Part model, mm, in its own coordinate system. A direction names the side the tool comes from. Give positions to 0.01 mm unless a question says otherwise; leave off trailing zeros. Order: outer loops, then holes, each group sorted by start corner. A loop starts at its lowest first (then second) coordinate and runs counter-clockwise, first axis right, second up.
1. Slice it at C-C on x = 0. Give the number of separate pieces and of enclosed holes in the cut face, and give its area (3 significant figures).
2. Slice it at D-D on z = -2. List the corners of the cut face in (x, y), and give its area (3 significant figures).
3. Slice it at B-B on y = 1. List the corners of the cut face in (x, z), and give its area (3 significant figures).
4. Mould opens along X. For faces 1 (the cylindrical face through (-1.29, -7.514, -2.024)), 2 (the flat face through (-16, 2, -4)), 3 (the cylindrical face through (-2.21, 2.03, -0.42)) say: +X half, -X half, draft (parallel to the pull), parting line (faces both ways), or undercut.
5. Slice it at A-A on z = -8. List the corners of the cut face in (x, y).
6. Probe line 1 (Z direction, x = 0, y = 5); line 2 (Y direction, x = -7, z = 2); line 3 (Z direction, x = 0, y = -6.75). List the from-to ranges inside material, lowest first.
7. Drop flat-ended pins along their axis: pin 1 Ø3 at (x, z) = (-23, -7.5) entering from +Y; pin 2 Ø6 at (y, z) = (-5.5, -4.5) entering from -X; pin 3 Ø6 at (x, z) = (2, -5.5) entering from +Y. Give the stop position or say it passes through.
8. Which spindle directions (+Z, -Z, +X, -X, +Y, -Y) get a long thin tool onto all of the face, cutting with end or side? Do faces 4 (the flat face through (-4, 0, 5)), 5 (the flat face through (-2, -6.5, 2)), 6 (the flat face through (0, 8.5, 2)), 7 (the flat face through (2, 6.5, 2)), 8 (the flat face through (-3, 3, -6)). Say none if no direction does.
from build123d import *

# Parameters (mm, degrees)
BOSS_EXTRUDE1_DEPTH            = 5
BOSS_EXTRUDE1_DEPTH_BACK       = 6
SKETCH2_R                      = 6
CUT_EXTRUDE1_REACH             = 14.01
SKETCH3_R                      = 3
CUT_EXTRUDE1_DIRECTION_2_REACH = 14.01
SKETCH4_R                      = 1.6
CUT_EXTRUDE4_DEPTH             = 17
BOSS_EXTRUDE2_DEPTH            = 2
BOSS_EXTRUDE2_DEPTH_BACK       = 2
SKETCH5_R                      = 1.35
FILLET1_R                      = 2
FILLET2_R                      = 1


with BuildPart() as part:
    # Sketch1 → Revolve1 (revolve)
    with BuildSketch(Plane.XY, mode=Mode.PRIVATE) as revolve1_sk:
        Polygon((1.6, -8.5), (1.6, 8.5), (2.4, 8.5), (2.4, 6.5), (4, 6.5), (4, -6.5), (2.4, -6.5), (2.4, -8.5), align=None)
    revolve(revolve1_sk.sketch.rotate(Axis((0, 9.772747413, 0), (0, -1, 0)), 180), axis=Axis((0, 9.772747413, 0), (0, -1, 0)))

    # Sketch2 → Boss-Extrude1 (add, two sides: drawn at the far end of the back side and taken through both)
    with BuildSketch(Plane.XY.offset(-BOSS_EXTRUDE1_DEPTH_BACK)):
        Circle(SKETCH2_R)
    extrude(amount=BOSS_EXTRUDE1_DEPTH + BOSS_EXTRUDE1_DEPTH_BACK)

    # Sketch3 → Cut-Extrude1 (cut, up to next)
    with BuildSketch(Plane.XY, mode=Mode.PRIVATE) as cut_extrude1_sk1:
        Circle(SKETCH3_R)
    cut_extrude1_tool1 = extrude(cut_extrude1_sk1.sketch, amount=-CUT_EXTRUDE1_REACH, mode=Mode.PRIVATE) & part.part
    add(cut_extrude1_tool1.solids().sort_by_distance((0, 0, 0))[0], mode=Mode.SUBTRACT)

    # Sketch3 → Cut-Extrude1 direction 2 (cut, up to next)
    with BuildSketch(Plane.XY, mode=Mode.PRIVATE) as cut_extrude1_direction_2_sk1:
        Circle(SKETCH3_R)
    cut_extrude1_direction_2_tool1 = extrude(cut_extrude1_direction_2_sk1.sketch, amount=CUT_EXTRUDE1_DIRECTION_2_REACH, mode=Mode.PRIVATE) & part.part
    add(cut_extrude1_direction_2_tool1.solids().sort_by_distance((0, 0, 0))[0], mode=Mode.SUBTRACT)

    # Sketch4 → Cut-Extrude4 (cut)
    with BuildSketch(Plane(origin=(0, 8.5, 0), x_dir=(1, 0, 0), z_dir=(0, 1, 0))):
        with Locations(Location((0, 0, 0), (0, 0, 180))):
            Circle(SKETCH4_R)
    extrude(amount=-CUT_EXTRUDE4_DEPTH, mode=Mode.SUBTRACT)

    # Sketch5 → Boss-Extrude2 (add, two sides: drawn at the far end of the back side and taken through both)
    with BuildSketch(Plane(origin=(0, 0, 0), x_dir=(1, 0, 0), z_dir=(0, 1, 0)).offset(-BOSS_EXTRUDE2_DEPTH_BACK)):
        with BuildLine():
            Line((-6, -5), (-10, -5))
            Line((-10, -5), (-25.5, 4))
            ThreePointArc((-25.5, 4), (-29.5, 8), (-25.5, 12))
            Line((-25.5, 12), (-23, 12))
            Line((-23, 12), (-8, 6))
            Line((-8, 6), (-6, 6))
            Line((-6, 6), (-3, 6))
            Line((-3, 6), (-3, -5))
            Line((-3, -5), (-6, -5))
        make_face()
        with Locations(Location((-25.5, 8, 0), (0, 0, 270))):
            Circle(SKETCH5_R, mode=Mode.SUBTRACT)
    extrude(amount=BOSS_EXTRUDE2_DEPTH + BOSS_EXTRUDE2_DEPTH_BACK)

    # Fillet1
    fillet1_edges = [part.edges().sort_by_distance(p)[0] for p in [
        (-5.656854249, 2, -0.5),
        (-5.656854249, -2, -0.5),
    ]]
    fillet(fillet1_edges, radius=FILLET1_R)

    # Fillet2
    fillet2_edges = [part.edges().sort_by_distance(p)[0] for p in [
        (-10, 0, 5),
        (-25.5, 0, -4),
        (-23, 0, -12),
        (-8, 0, -6),
    ]]
    fillet(fillet2_edges, radius=FILLET2_R)


solid = part.part
Data:
1. separate pieces: 4
1. enclosed holes: 0
1. area: 58.0 mm2
2. outline: (-22.06, -2) - (-6.93, -2) arc R2 cw to (-5.2, -3) arc R6 ccw to (-3.46, -4.9) - (-3.46, -6.5) - (-1.33, -6.5) - (-1.33, -8.5) - (1.33, -8.5) - (1.33, -6.5) - (3.46, -6.5) - (3.46, -4.9) arc R6 ccw to (3.46, 4.9) - (3.46, 6.5) - (1.33, 6.5) - (1.33, 8.5) - (-1.33, 8.5) - (-1.33, 6.5) - (-3.46, 6.5) - (-3.46, 4.9) arc R6 ccw to (-5.2, 3) arc R2 cw to (-6.93, 2) - (-22.06, 2) - close; hole circle Ø6 at (0, 0)
2. area: 172 mm2
3. outline: (-25.73, -4.01) arc R4 ccw to (-25.5, -12) - (-23.19, -12) arc R1 ccw to (-22.82, -11.93) - (-8.18, -6.07) arc R1 cw to (-7.81, -6) - (-2.83, -6) - (-2.83, 5) - (-9.73, 5) arc R1 ccw to (-10.23, 4.86) - (-25.28, -3.87) arc R1 cw to start; (2.83, -6) - (5.92, -6) - (5.92, 5) - (2.83, 5) - close; hole circle Ø2.7 at (-25.5, -8)
3. area: 293 mm2
4. face 1: parting line
4. face 2: draft
4. face 3: undercut
5. outline: (-29.5, -2) - (-26.85, -2) - (-26.85, 2) - (-29.5, 2) - close; (-24.15, -2) - (-13, -2) - (-13, 2) - (-24.15, 2) - close
6. line 1: z = -6 to -1.6, 1.6 to 5
6. line 2: y = -2 to 2
6. line 3: z = -2.4 to -1.6, 1.6 to 2.4
7. pin 1: stops at y = 2
7. pin 2: stops at x = -5.61
7. pin 3: stops at y = 6.5
8. face 4: +Z, +X, -X, +Y, -Y
8. face 5: -Y
8. face 6: +Z, -Z, +X, -X, +Y
8. face 7: +Y
8. face 8: -Z, +X, +Y, -Y
